For this review, take the finished solid that the model builds, in its own axes (mm). Face numbers are marked on the shaded views. A direction names the side the tool comes from. Round coordinates to 2 decimals unless told otherwise and drop trailing zeros. Loops run counter-clockwise (first coordinate to the right, second up) from the corner with the lowest first, then second, coordinate; pieces in that order, holes last.
1. Draft analysis for pull direction Z (two halves, no side actions). For the marked faces 1, 2 and 3, state which applies: released by +Z, released by -Z, zero draft, split by the parting line, or undercut.
2. Tool access review of the marked faces 4, 5 and 6: name each direction out of +Z, -Z, +X, -X, +Y, -Y from which nothing blocks a thin tool from reaching the whole face with its end or side.
3. Consider section C-C on y = 25. State the section outline as (x, z) points.
4. Consider section A-A on x = -75. State the section outline as (y, z) points, then the cut area to 3 significant figures.
5. To check wall thickness, follow line 1 along Y through (x, z) = (-75, 17); line 2 along Z through (x, y) = (1, -39); line 3 along Y through (x, z) = (-5, -2). State the ranges of each line that lie inside material, in increasing order.
6. Clearance check with flat-ended pins moving along their axes: pin 1 Ø8 at (x, z) = (30, -12.5) entering from +Y; pin 2 Ø10.5 at (x, z) = (-43, 14) entering from +Y; pin 3 Ø12 at (x, y) = (-65.5, 19.5) entering from -Z; pin 4 Ø12.5 at (x, y) = (75, -45) entering from +Z. State where each tip first meets the part, or that it passes through.
7. Consider section D-D on z = -10.5. State the section outline as (x, y) points.
8. Consider section B-B on y = 45. State the section outline as (x, z) points.
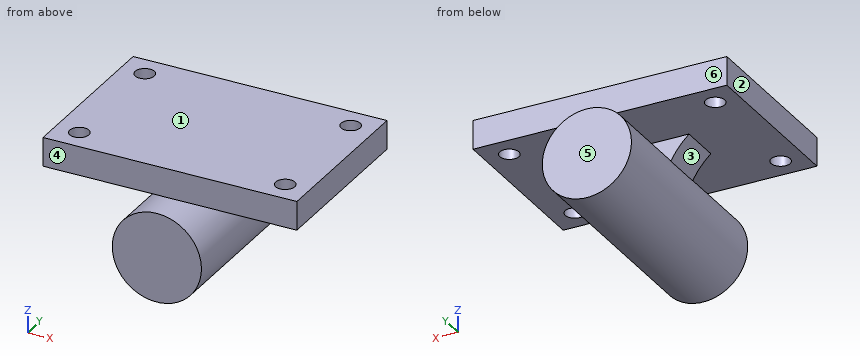
from build123d import *

# Parameters (mm, degrees)
SKETCH_1_W          = 185
SKETCH_1_H          = 124
EXTRUDE_1_DEPTH     = 21
EXTRUDE_2_DEPTH     = 15
SKETCH_5_R          = 32.5
EXTRUDE_3_DEPTH     = 80
SKETCH_6_R          = 7
CUT_EXTRUDE_1_DEPTH = 140.687150447


with BuildPart() as part:
    # 草图1 → 凸台-拉伸1 (new body)
    with BuildSketch(Plane.XY):
        Rectangle(SKETCH_1_W, SKETCH_1_H)
    extrude(amount=EXTRUDE_1_DEPTH)

    # 草图3 → 凸台-拉伸2 (add, symmetric)
    with BuildSketch(Plane(origin=(0, 0, 0), x_dir=(1, 0, 0), z_dir=(0, 1, 0))):
        with BuildLine():
            Line((40, 0), (-40, 0))
            ThreePointArc((-40, 0), (-26.459601843, 16.925451065), (-19.835033499, 37.563483197))
            ThreePointArc((-19.835033499, 37.563483197), (0, 15), (19.835033499, 37.563483197))
            ThreePointArc((19.835033499, 37.563483197), (26.459601843, 16.925451065), (40, 0))
        make_face()
    extrude(amount=EXTRUDE_2_DEPTH, both=True)

    # 草图5 → 凸台-拉伸3 (add, symmetric)
    with BuildSketch(Plane(origin=(0, 0, 0), x_dir=(1, 0, 0), z_dir=(0, 1, 0))):
        with Locations(Location((0, 35, 0), (0, 0, 270))):
            Circle(SKETCH_5_R)
    extrude(amount=EXTRUDE_3_DEPTH, both=True)

    # 草图6 → 切除-拉伸1 (cut, through all)
    with BuildSketch(Plane(origin=(0, 0, 0), x_dir=(-1, 0, 0), z_dir=(0, 0, -1))):
        with Locations((-75, 45)):
            Circle(SKETCH_6_R)
        with Locations((75, 45)):
            Circle(SKETCH_6_R)
        with Locations((75, -45)):
            Circle(SKETCH_6_R)
        with Locations((-75, -45)):
            Circle(SKETCH_6_R)
    extrude(amount=-CUT_EXTRUDE_1_DEPTH, mode=Mode.SUBTRACT)


solid = part.part
Resolved:
1. face 1: released by +Z
1. face 2: zero draft
1. face 3: undercut
2. face 4: +Z, +X, -X, -Y
2. face 5: +Z, -Z, +X, -X, +Y
2. face 6: +Z, +X, -X, +Y
3. outline: (-92.5, 0) - (92.5, 0) - (92.5, 21) - (-92.5, 21) - close; circle Ø65 at (0, -35)
4. outline: (-62, 0) - (-52, 0) - (-52, 21) - (-62, 21) - close; (-38, 0) - (38, 0) - (38, 21) - (-38, 21) - close; (52, 0) - (62, 0) - (62, 21) - (52, 21) - close
4. area: 2,020 mm2
5. line 1: y = -62 to -52, -38 to 38, 52 to 62
5. line 2: z = -67.48 to -2.52, 0 to 21
5. line 3: y = -15 to 15
6. pin 1: stops at y = 15
6. pin 2: stops at y = 62
6. pin 3: stops at z = 0
6. pin 4: passes through
7. outline: (-30.45, -15) - (-21.35, -15) - (-21.35, -80) - (21.35, -80) - (21.35, -15) - (30.45, -15) - (30.45, 15) - (21.35, 15) - (21.35, 80) - (-21.35, 80) - (-21.35, 15) - (-30.45, 15) - close
8. outline: (-92.5, 0) - (-82, 0) - (-82, 21) - (-92.5, 21) - close; (-68, 0) - (68, 0) - (68, 21) - (-68, 21) - close; circle Ø65 at (0, -35); (82, 0) - (92.5, 0) - (92.5, 21) - (82, 21) - close
